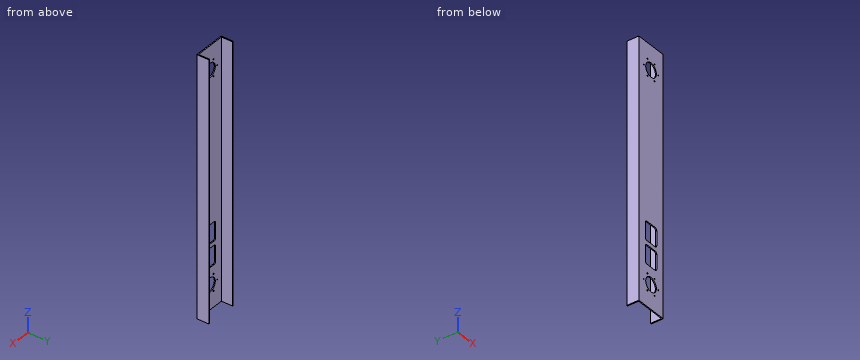
```python
from build123d import *

# Parameters (mm, degrees)
BOSS_EXTRUDE1_DEPTH = 812.8
SKETCH2_R           = 22.2377
CUT_EXTRUDE1_DEPTH  = 3.175
SKETCH3_R           = 1.89865
CUT_EXTRUDE2_DEPTH  = 3.175
CUT_EXTRUDE3_REACH  = 40.1


with BuildPart() as part:
    # Sketch1 → Boss-Extrude1 (new body)
    with BuildSketch(Plane.XY):
        Polygon((3.175, 3.175), (3.175, 38.1), (0, 38.1), (0, 0), (101.6, 0), (101.6, 38.1), (98.425, 38.1), (98.425, 3.175), align=None)
    extrude(amount=BOSS_EXTRUDE1_DEPTH)

    # Sketch2 → Cut-Extrude1 (cut)
    with BuildSketch(Plane.XZ):
        with Locations((50.8, 736.6)):
            Circle(SKETCH2_R)
    cut_extrude1 = extrude(amount=-CUT_EXTRUDE1_DEPTH, mode=Mode.SUBTRACT)

    # Sketch3 → Cut-Extrude2 (cut)
    with BuildSketch(Plane.XZ):
        with Locations((65.88125, 762.721491242)):
            Circle(SKETCH3_R)
        with Locations((80.9625, 736.6)):
            Circle(SKETCH3_R)
        with Locations((65.88125, 710.478508758)):
            Circle(SKETCH3_R)
        with Locations((35.71875, 710.478508758)):
            Circle(SKETCH3_R)
        with Locations((20.6375, 736.6)):
            Circle(SKETCH3_R)
        with Locations((35.71875, 762.721491242)):
            Circle(SKETCH3_R)
    cut_extrude2 = extrude(amount=-CUT_EXTRUDE2_DEPTH, mode=Mode.SUBTRACT)

    # Mirror1: Cut-Extrude1, Cut-Extrude2 across plane
    add(cut_extrude1.mirror(Plane.XY.offset(406.4)), mode=Mode.SUBTRACT)
    add(cut_extrude2.mirror(Plane.XY.offset(406.4)), mode=Mode.SUBTRACT)

    # Sketch4 → Cut-Extrude3 (cut, up to next)
    with BuildSketch(Plane.XZ, mode=Mode.PRIVATE) as cut_extrude3_sk1:
        with BuildLine():
            Line((68.2625, 129.836281806), (33.3375, 129.836281806))
            ThreePointArc((33.3375, 129.836281806), (28.847371939, 131.696153745), (26.9875, 136.186281806))
            Line((26.9875, 136.186281806), (26.9875, 183.200007549))
            ThreePointArc((26.9875, 183.200007549), (28.847371939, 187.690135609), (33.3375, 189.550007549))
            Line((33.3375, 189.550007549), (68.2625, 189.550007549))
            ThreePointArc((68.2625, 189.550007549), (72.752628061, 187.690135609), (74.6125, 183.200007549))
            Line((74.6125, 183.200007549), (74.6125, 136.186281806))
            ThreePointArc((74.6125, 136.186281806), (72.752628061, 131.696153745), (68.2625, 129.836281806))
        make_face()
    cut_extrude3_tool1 = extrude(cut_extrude3_sk1.sketch, amount=-CUT_EXTRUDE3_REACH, mode=Mode.PRIVATE) & part.part
    add(cut_extrude3_tool1.solids().sort_by_distance((50.8, 0, 159.693145))[0], mode=Mode.SUBTRACT)
    # Sketch4 → Cut-Extrude3 (cut, up to next)
    with BuildSketch(Plane.XZ, mode=Mode.PRIVATE) as cut_extrude3_sk2:
        with BuildLine():
            Line((68.2625, 261.963733292), (33.3375, 261.963733292))
            ThreePointArc((33.3375, 261.963733292), (28.847371939, 260.103861353), (26.9875, 255.613733292))
            Line((26.9875, 255.613733292), (26.9875, 208.600007549))
            ThreePointArc((26.9875, 208.600007549), (28.847371939, 204.109879488), (33.3375, 202.250007549))
            Line((33.3375, 202.250007549), (68.2625, 202.250007549))
            ThreePointArc((68.2625, 202.250007549), (72.752628061, 204.109879488), (74.6125, 208.600007549))
            Line((74.6125, 208.600007549), (74.6125, 255.613733292))
            ThreePointArc((74.6125, 255.613733292), (72.752628061, 260.103861353), (68.2625, 261.963733292))
        make_face()
    cut_extrude3_tool2 = extrude(cut_extrude3_sk2.sketch, amount=-CUT_EXTRUDE3_REACH, mode=Mode.PRIVATE) & part.part
    add(cut_extrude3_tool2.solids().sort_by_distance((50.8, 0, 232.10687))[0], mode=Mode.SUBTRACT)


solid = part.part
```
Check sheet for the modelled part. Datum: model origin and axes. Units: mm. Coordinates: 2 decimals unless noted, no trailing zeros. Loops run counter-clockwise (first coordinate to the right, second up) from the corner with the lowest first, then second, coordinate; pieces in that order, holes last.
1) Gauge pin test, flat ends, axial feed: pin 1 (4.5 mm diameter, centred on x = 65.88, z = 710.48, fed in from -Y); pin 2 (3 mm diameter, centred on x = 80.96, z = 76.2, fed in from +Y); pin 3 (5 mm diameter, centred on x = 35.72, z = 50.08, fed in from +Y) (3 decimals). Record the tip position at first contact, or that the pin passes through.
2) Sectioned sample at B-B (y = 23.5). Record the boundary of the cut face in (x, z) (3 decimals).
3) Material ranges on probe 1 along X at (y, z) = (13, 54) (3 decimals); probe 2 along Y at (x, z) = (8, 50) (3 decimals), recorded low to high.
4) Sectioned sample at A-A (x = 50.8). Record the boundary of the cut face in (y, z) (3 decimals), and give its area (3 significant figures).
5) Sectioned sample at C-C (z = 237). Record the boundary of the cut face in (x, y) (1 decimal), and give its area (3 significant figures).
6) Sectioned sample at D-D (z = 586.5). Record the boundary of the cut face in (x, y) (3 decimals), and give its area (3 significant figures).
Check sheet entries:
1. pin 1: stops at y = 0
1. pin 2: passes through
1. pin 3: stops at y = 3.175
2. outline: (0, 0) - (3.175, 0) - (3.175, 812.8) - (0, 812.8) - close; (98.425, 0) - (101.6, 0) - (101.6, 812.8) - (98.425, 812.8) - close
3. probe 1: x = 0 to 3.175, 98.425 to 101.6
3. probe 2: y = 0 to 3.175
4. outline: (0, 0) - (3.175, 0) - (3.175, 53.962) - (0, 53.962) - close; (0, 98.438) - (3.175, 98.438) - (3.175, 129.836) - (0, 129.836) - close; (0, 189.55) - (3.175, 189.55) - (3.175, 202.25) - (0, 202.25) - close; (0, 261.964) - (3.175, 261.964) - (3.175, 714.362) - (0, 714.362) - close; (0, 758.838) - (3.175, 758.838) - (3.175, 812.8) - (0, 812.8) - close
4. area: 1,920 mm2
5. outline: (0, 0) - (27, 0) - (27, 3.2) - (3.2, 3.2) - (3.2, 38.1) - (0, 38.1) - close; (74.6, 0) - (101.6, 0) - (101.6, 38.1) - (98.4, 38.1) - (98.4, 3.2) - (74.6, 3.2) - close
5. area: 393 mm2
6. outline: (0, 0) - (101.6, 0) - (101.6, 38.1) - (98.425, 38.1) - (98.425, 3.175) - (3.175, 3.175) - (3.175, 38.1) - (0, 38.1) - close
6. area: 544 mm2
